Can you work these out from the model? Positions are in its coordinate system, mm. Give positions to 0.01 mm unless a question says otherwise; leave off trailing zeros. Put each result on its own line as item: value. Start each with the question number.
1) Imagine slicing it at A-A (z = 6.75). State how many separate pieces and enclosed holes the cut face has, then the cut area to 3 significant figures.
2) For P1, Ø5, axis at x = 2, y = -381.5, coming from the +Z side, with a flat end and sliding along its axis, tell me the tip position at first contact or that it passes through.
3) Please list where these lines run through material, in increasing order: line 1 along X through (y, z) = (-103, 1.25) (3 decimals); line 2 along X through (y, z) = (-173.5, 2.5) (1 decimal); line 3 along Z through (x, y) = (8, -128). Write a range as from..to.
from build123d import *

# Parameters (mm, degrees)
F1_DEPTH = 609.6
F2_SIZE  = 1.5875
F5_W     = 34.925
F5_H     = 12.7
F6_DEPTH = 609.601


with BuildPart() as f1:
    # F0 (on Front) → F1 (new body)
    with BuildSketch(Plane.XZ):
        Polygon((0, 1.5875), (0, 0), (10.31875, 0), (10.31875, 1.5875), (7.9375, 1.5875), (7.9375, 11.1125), (14.2875, 11.1125), (14.2875, 12.7), (3.96875, 12.7), (3.96875, 11.1125), (6.35, 11.1125), (6.35, 1.5875), align=None)
    extrude(amount=F1_DEPTH)

    # F2
    f2_edges = [f1.edges().sort_by_distance(p)[0] for p in [
        (6.35, -304.8, 1.5875),
        (7.9375, -304.8, 11.1125),
    ]]
    chamfer(f2_edges, length=F2_SIZE)

    # F3: F1 across face


with BuildPart() as f1_1:
    add(f1.part)
    add(f1.part.mirror(Plane(origin=(14.2875, -304.8, 11.90625), x_dir=(0, 1, 0), z_dir=(1, 0, 0))))

    # F4: F1 across face


with BuildPart() as f1_2:
    add(f1_1.part)
    add(f1_1.part.mirror(Plane(origin=(28.575, -304.8, 0.79375), x_dir=(0, 1, 0), z_dir=(1, 0, 0))))

    # F5 (on face) → F6 (cut, through all)
    with BuildSketch(Plane.XZ.offset(609.6)):
        with Locations((39.6875, 6.35)):
            Rectangle(F5_W, F5_H)
    extrude(amount=-F6_DEPTH, mode=Mode.SUBTRACT)

    # F7: F1 across face


with BuildPart() as f1_3:
    add(f1_2.part)
    add(f1_2.part.mirror(Plane(origin=(0, -304.8, 0.79375), x_dir=(0, -1, 0), z_dir=(-1, 0, 0))))


solid = f1_3.part
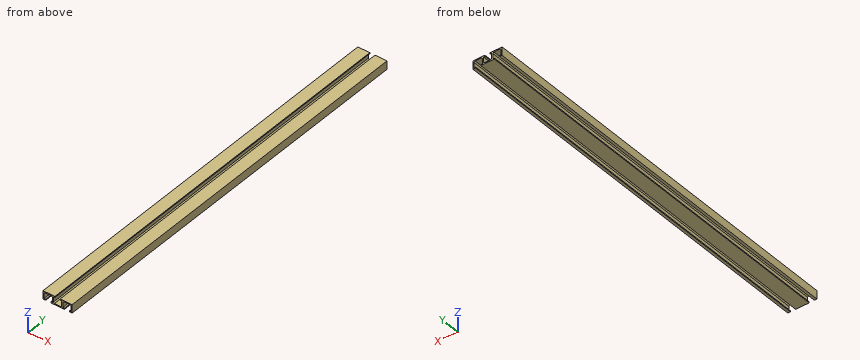
Recorded:
1. separate pieces: 4
1. enclosed holes: 0
1. area: 3,870 mm²
2. P1: z = 12.7
3. line 1: -22.225..-18.256, -10.319..10.319, 18.256..22.225
3. line 2: -22.2..-20.6, -7.9..-5.7, 5.7..7.9, 20.6..22.2
3. line 3: 0..1.59, 9.59..12.7
